Verification items for the finished model (mm, model axes). Face numbers are marked on the shaded views. A direction names the side the tool comes from. Round coordinates to 2 decimals unless told otherwise and drop trailing zeros. Write each loop counter-clockwise with the first axis right and the second up, starting at its lowest first coordinate (ties: lowest second). Pieces come first, ordered by that corner, then holes. Notation, with made-up numbers: (37.25, 69.5) - (61.25, 69.5) arc R17 ccw to (61.25, 85.5) - close; hole circle Ø6 at (-39.5, 39.5). An arc over 180 degrees is marked (long way). Answer as a JSON object with one key per item and string values.
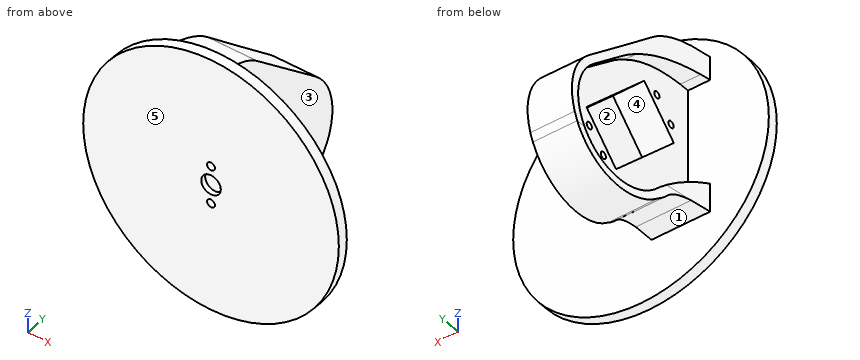
```python
from build123d import *

# Parameters (mm, degrees)
CROQUIS1_R                 = 49
SALIENTE_EXTRUIR1_DEPTH    = 4
CROQUIS2_R                 = 1.5
CORTAR_EXTRUIR1_DEPTH      = 4
CROQUIS3_W                 = 22.5
CROQUIS3_H                 = 60.679
SALIENTE_EXTRUIR2_DEPTH    = 60.773
SALIENTE_EXTRUIR3_DEPTH    = 22.5
CORTAR_EXTRUIR2_DEPTH      = 22.5
CORTAR_EXTRUIR5_DEPTH      = 8.5
CORTAR_EXTRUIR6_DEPTH      = 29.5
CORTAR_EXTRUIR6_DEPTH_BACK = 78.5
CORTAR_EXTRUIR7_DEPTH      = 12
CORTAR_EXTRUIR8_REACH      = 57
CROQUIS12_R                = 9
CROQUIS13_R                = 1.3
CORTAR_EXTRUIR9_DEPTH      = 5
CROQUIS14_R                = 3.75
CORTAR_EXTRUIR10_DEPTH     = 2


with BuildPart() as part:
    # Croquis1 → Saliente-Extruir1 (new body)
    with BuildSketch(Plane(origin=(0, 0, 0), x_dir=(1, 0, 0), z_dir=(0, 1, 0))):
        Circle(CROQUIS1_R)
    extrude(amount=SALIENTE_EXTRUIR1_DEPTH)

    # Croquis2 → Cortar-Extruir1 (cut)
    with BuildSketch(Plane(origin=(0, 4, 0), x_dir=(1, 0, 0), z_dir=(0, 1, 0))):
        with Locations((0, 7.25)):
            Circle(CROQUIS2_R)
        with Locations((0, -7.25)):
            Circle(CROQUIS2_R)
    extrude(amount=-CORTAR_EXTRUIR1_DEPTH, mode=Mode.SUBTRACT)

    # Croquis3 → Saliente-Extruir2 (add)
    with BuildSketch(Plane(origin=(0, 4, 0), x_dir=(1, 0, 0), z_dir=(0, 1, 0))):
        with Locations((-15.25, -4.2105)):
            Rectangle(CROQUIS3_W, CROQUIS3_H)
    extrude(amount=SALIENTE_EXTRUIR2_DEPTH)

    # Croquis4 → Saliente-Extruir3 (add)
    with BuildSketch(Plane(origin=(-4, 0, 0), x_dir=(0, 0, -1), z_dir=(1, 0, 0))):
        with BuildLine():
            Line((-34.55, 4), (-34.55, 11.858))
            add(Edge.make_bspline(
                [(-34.55, 11.858), (-34.026556698, 21.514345964), (-28.575, 28.098)],
                knots=[0, 0, 0, 0.824435894, 0.824435894, 0.824435894], degree=2))
            Line((-28.575, 28.098), (-3.407, 57.621))
            ThreePointArc((-3.407, 57.621), (30.992681607, 60.270900315), (33.465, 25.858))
            add(Edge.make_bspline(
                [(29.748, 21.629), (31.899002628, 23.543234873), (33.465, 25.858)],
                knots=[0, 0, 0, 0.522921898, 0.522921898, 0.522921898], degree=2))
            add(Edge.make_bspline(
                [(26.129, 11.858), (26.849165043, 18.857512826), (29.748, 21.629)],
                knots=[0, 0, 0, 0.117772871, 0.117772871, 0.117772871], degree=2))
            Line((26.129, 11.858), (26.129, 4))
            Line((26.129, 4), (-34.55, 4))
        make_face()
    extrude(amount=-SALIENTE_EXTRUIR3_DEPTH)

    # Croquis5 → Cortar-Extruir2 (cut)
    with BuildSketch(Plane(origin=(-4, 0, 0), x_dir=(0, 0, -1), z_dir=(1, 0, 0))):
        with BuildLine():
            Line((-27.985060499, 28.790020974), (-3.407, 57.621))
            ThreePointArc((-3.407, 57.621), (1.319630754, 61.88266891), (6.989626025, 64.773))
            Line((6.989626025, 64.773), (-34.55, 64.773))
            Line((-34.55, 64.773), (-34.55, 11.858))
            add(Edge.make_bspline(
                [(-34.55, 11.858), (-34.095195054, 18.386707566), (-32.103528387, 23.800040899), (-28.575, 28.098)],
                knots=[0, 0, 0, 0, 0.605648705, 0.605648705, 0.605648705, 0.605648705], degree=3))
            add(Edge.make_bspline(
                [(-28.575, 28.098), (-28.382908254, 28.331979262), (-28.186261754, 28.56265292), (-27.985060499, 28.790020974)],
                knots=[0.605648705, 0.605648705, 0.605648705, 0.605648705, 0.638619991, 0.638619991, 0.638619991, 0.638619991], degree=3))
        make_face()
        with BuildLine():
            ThreePointArc((23.232314116, 64.773), (24.700788316, 64.198896251), (26.129, 63.530897014))
            Line((26.129, 63.530897014), (26.129, 64.773))
            Line((26.129, 64.773), (23.232314116, 64.773))
        make_face()
    extrude(amount=-CORTAR_EXTRUIR2_DEPTH, mode=Mode.SUBTRACT)

    # Croquis9 → Cortar-Extruir5 (cut)
    with BuildSketch(Plane.ZY.offset(26.5)):
        with BuildLine():
            Line((25.55, 4), (25.55, 7.838))
            add(Edge.make_bspline(
                [(25.55, 7.838), (24.886302853, 23.956871559), (17.259, 35.7)],
                knots=[0, 0, 0, 0.526933163, 0.526933163, 0.526933163], degree=2))
            add(Edge.make_bspline(
                [(17.259, 35.7), (14.834185302, 39.750302487), (11.753, 43.195)],
                knots=[0, 0, 0, 0.431108937, 0.431108937, 0.431108937], degree=2))
            Line((11.753, 43.195), (1.123987272, 55.674759295))
            ThreePointArc((1.123987272, 55.674759295), (-28.963418372, 57.90340371), (-31.192062787, 27.815998066))
            add(Edge.make_bspline(
                [(-15.129, 4), (-20.706034624, 17.629178957), (-31.192062787, 27.815998066)],
                knots=[0, 0, 0, 1, 1, 1], degree=2))
            Line((-15.129, 4), (25.55, 4))
        make_face()
    extrude(amount=-CORTAR_EXTRUIR5_DEPTH, mode=Mode.SUBTRACT)

    # Croquis10 → Cortar-Extruir6 (cut, two sides)
    with BuildSketch(Plane(origin=(0, 0, -26.129), x_dir=(-1, 0, 0), z_dir=(0, 0, -1))) as cortar_extruir6_sk:
        with BuildLine():
            Line((21, 66.168251112), (26.5, 66.168251112))
            Line((26.5, 66.168251112), (26.5, 4))
            add(Edge.make_bspline(
                [(21, 66.168251112), (21.140868098, 34.670825733), (26.5, 4)],
                knots=[0, 0, 0, 0.615166298, 0.615166298, 0.615166298], degree=2))
        make_face()
    extrude(amount=CORTAR_EXTRUIR6_DEPTH, mode=Mode.SUBTRACT)
    extrude(cortar_extruir6_sk.sketch, amount=-CORTAR_EXTRUIR6_DEPTH_BACK, mode=Mode.SUBTRACT)

    # Croquis11 → Cortar-Extruir7 (cut)
    with BuildSketch(Plane.ZY.offset(18)):
        Polygon((0.401, 11.108), (15.25, 25.957), (-13.741, 54.948), (-28.59, 40.099), align=None)
    extrude(amount=-CORTAR_EXTRUIR7_DEPTH, mode=Mode.SUBTRACT)

    # Croquis12 → Cortar-Extruir8 (cut, up to next)
    with BuildSketch(Plane.ZY.offset(6), mode=Mode.PRIVATE) as cortar_extruir8_sk1:
        with Locations((-13.918, 40.276)):
            Circle(CROQUIS12_R)
    cortar_extruir8_tool1 = extrude(cortar_extruir8_sk1.sketch, amount=-CORTAR_EXTRUIR8_REACH, mode=Mode.PRIVATE) & part.part
    add(cortar_extruir8_tool1.solids().sort_by_distance((-6, 40.276, -13.918))[0], mode=Mode.SUBTRACT)

    # Croquis13 → Cortar-Extruir9 (cut)
    with BuildSketch(Plane.ZY.offset(18)):
        with Locations((-27.176836773, 46.464011366)):
            Circle(CROQUIS13_R)
        with Locations((-20.104694437, 53.533519844)):
            Circle(CROQUIS13_R)
        with Locations((6.766011366, 12.521163227)):
            Circle(CROQUIS13_R)
        with Locations((13.836836773, 19.591988634)):
            Circle(CROQUIS13_R)
    extrude(amount=-CORTAR_EXTRUIR9_DEPTH, mode=Mode.SUBTRACT)

    # Croquis14 → Cortar-Extruir10 (cut)
    with BuildSketch(Plane.XZ):
        Circle(CROQUIS14_R)
    extrude(amount=-CORTAR_EXTRUIR10_DEPTH, mode=Mode.SUBTRACT)


solid = part.part
```
1. Material ranges on probe 1 along Y at (x, z) = (-29, 11.5); probe 2 along X at (y, z) = (2, 7); probe 3 along X at (y, z) = (40.5, 11.5), recorded low to high. Write a range as from..to.
Completed:
{"probe 1": "y = 0..4", "probe 2": "x = -48.5..-1.48, 1.48..48.5", "probe 3": "x = -18..-4"}
2. Cross-section at C-C (z = 41.5). Record the boundary of the cut face in (x, y).
Completed:
{"outline": "(-26.05, 0) - (26.05, 0) - (26.05, 4) - (-26.05, 4) - close"}
3. Cross-section at B-B (z = -7.25). Count the separate pieces of the cut face and the enclosed holes in it, plus the area to 3 significant figures.
Completed:
{"separate pieces": "3", "enclosed holes": "0", "area": "857 mm^2"}
4. Mould release check, pull along Y, two halves, no side actions. Record for the marked faces 3, 4 and 5: released by +Y, released by -Y, zero draft, split by the parting line, or undercut.
Completed:
{"face 3": "zero draft", "face 4": "undercut", "face 5": "released by -Y"}
5. Go/stop test with flat-tipped pins: pin 1 (22 mm diameter, centred on y = 30, z = -2.5, fed in from -X); pin 2 (1.3 mm diameter, centred on y = 13, z = 7, fed in from -X); pin 3 (3 mm diameter, centred on y = 12.52, z = 6.77, fed in from +X). Record where each tip stops, or that it passes through.
Completed:
{"pin 1": "stops at x = -18", "pin 2": "stops at x = -13", "pin 3": "stops at x = -4"}
6. Access from +Z, -Z, +X, -X, +Y, -Y to the whole of each face (thin tool, end or side, straight path). Record for the marked faces 1 and 2.
Completed:
{"face 1": "-Z, +X, -X", "face 2": "-X"}
7. Cross-section at A-A (x = 0). Record the boundary of the cut face in (y, z).
Completed:
{"outline": "(0, -49) - (4, -49) - (4, -8.75) - (0, -8.75) - close; (0, -5.75) - (4, -5.75) - (4, 5.75) - (0, 5.75) - (0, 3.75) - (2, 3.75) - (2, -3.75) - (0, -3.75) - close; (0, 8.75) - (4, 8.75) - (4, 49) - (0, 49) - close"}
